Here's how the part is built. I have some questions about the finished solid (model axes, mm). Coordinates: 2 decimals unless noted, no trailing zeros. Write each loop counter-clockwise with the first axis right and the second up, starting at its lowest first coordinate (ties: lowest second). Pieces come first, ordered by that corner, then holes.
(1) Imagine slicing it at D-D, the plane z = 0.7. List the corners of the cut face in (x, y) for me, plus the area to 3 significant figures.
(2) Imagine slicing it at C-C, the plane y = -16.5. List the corners of the cut face in (x, z) for me.
(3) Please list where these lines run through material, in increasing order: probe 1 along Y at (x, z) = (0, 1.8); probe 2 along X at (y, z) = (-19, 2.3); probe 3 along X at (y, z) = (14, 1.7).
(4) Imagine slicing it at A-A, the plane y = 0. List the corners of the cut face in (x, z) for me, plus the area to 3 significant figures.
(5) Thinking about a two-plate mould opening in Y: for faces 1 (the flat face through (28, 1, 3)), 2 (the cylindrical face through (-5.598, 42.634, 1.479)), 3 (the cylindrical face through (-25.81, -17.65, 1.48)), which applies, released by +Y, released by -Y, zero draft, split by the parting line, or undercut?
(6) For pin 1 Ø5.5 at (x, y) = (-28.58, -16.5) entering from -Z; pin 2 Ø1 at (y, z) = (-23, 2) entering from -X; pin 3 Ø1 at (x, z) = (4, 1) entering from -Y, each with a flat end and sliding along its axis, tell me the tip position at first contact or that it passes through.
(7) Imagine slicing it at B-B, the plane x = 0. List the corners of the cut face in (y, z) for me, plus the area to 3 significant figures.
```python
from build123d import *

# Parameters (mm, degrees)
SKETCH1_R           = 43
BOSS_EXTRUDE2_DEPTH = 3
SKETCH1_3_R         = 3
CUT_EXTRUDE1_DEPTH  = 4
CIRPATTERN2_COUNT   = 6
SKETCH1_4_R         = 27.5
CUT_EXTRUDE2_DEPTH  = 4


with BuildPart() as part:
    # Sketch1 → Boss-Extrude2 (new body)
    with BuildSketch(Plane.XY):
        Circle(SKETCH1_R)
    extrude(amount=BOSS_EXTRUDE2_DEPTH)

    # Sketch1_3 → Cut-Extrude1 (cut, through all)
    with BuildSketch(Plane.XY):
        with Locations((0, 33)):
            Circle(SKETCH1_3_R)
    cut_extrude1 = extrude(amount=CUT_EXTRUDE1_DEPTH, mode=Mode.SUBTRACT)

    # CirPattern2: Cut-Extrude1 ×6 about axis
    cirpattern2_axis = Axis((0, 0, 0), (0, 0, 1))
    for i in range(1, CIRPATTERN2_COUNT):
        add(cut_extrude1.rotate(cirpattern2_axis, i * 360 / CIRPATTERN2_COUNT), mode=Mode.SUBTRACT)

    # Sketch1_4 → Cut-Extrude2 (cut, through all)
    with BuildSketch(Plane.XY):
        Circle(SKETCH1_4_R)
    extrude(amount=CUT_EXTRUDE2_DEPTH, mode=Mode.SUBTRACT)


solid = part.part
```
Recorded:
1. outline: circle Ø86 at (0, 0); hole circle Ø6 at (-28.58, -16.5); hole circle Ø6 at (-28.58, 16.5); hole circle Ø55 at (0, 0); hole circle Ø6 at (0, -33); hole circle Ø6 at (0, 33); hole circle Ø6 at (28.58, -16.5); hole circle Ø6 at (28.58, 16.5)
1. area: 3,260 mm2
2. outline: (-39.71, 0) - (-31.58, 0) - (-31.58, 3) - (-39.71, 3) - close; (-25.58, 0) - (-22, 0) - (-22, 3) - (-25.58, 3) - close; (22, 0) - (25.58, 0) - (25.58, 3) - (22, 3) - close; (31.58, 0) - (39.71, 0) - (39.71, 3) - (31.58, 3) - close
3. probe 1: y = -43 to -36, -30 to -27.5, 27.5 to 30, 36 to 43
3. probe 2: x = -38.57 to -30.24, -26.92 to -19.88, 19.88 to 26.92, 30.24 to 38.57
3. probe 3: x = -40.66 to -30.24, -26.92 to -23.67, 23.67 to 26.92, 30.24 to 40.66
4. outline: (-43, 0) - (-27.5, 0) - (-27.5, 3) - (-43, 3) - close; (27.5, 0) - (43, 0) - (43, 3) - (27.5, 3) - close
4. area: 93.0 mm2
5. face 1: zero draft
5. face 2: split by the parting line
5. face 3: undercut
6. pin 1: passes through
6. pin 2: stops at x = -36.64
6. pin 3: stops at y = -42.86
7. outline: (-43, 0) - (-36, 0) - (-36, 3) - (-43, 3) - close; (-30, 0) - (-27.5, 0) - (-27.5, 3) - (-30, 3) - close; (27.5, 0) - (30, 0) - (30, 3) - (27.5, 3) - close; (36, 0) - (43, 0) - (43, 3) - (36, 3) - close
7. area: 57.0 mm2
